```python
from build123d import *

# Parameters (mm, degrees)
SKETCH1_W           = 17
SKETCH1_H           = 30
BOSS_EXTRUDE1_DEPTH = 3
SKETCH2_W           = 3
SKETCH2_H           = 5
CUT_EXTRUDE1_DEPTH  = 3
SKETCH3_R           = 1.5
CUT_EXTRUDE2_DEPTH  = 3
FILLET1_R           = 3
SKETCH4_W           = 30
SKETCH4_H           = 30
BOSS_EXTRUDE2_DEPTH = 3
FILLET2_R           = 3
SKETCH5_R           = 2
CUT_EXTRUDE3_DEPTH  = 3
SKETCH6_W           = 3
SKETCH6_H           = 3
CUT_EXTRUDE4_DEPTH  = 10


with BuildPart() as part:
    # Sketch1 → Boss-Extrude1 (new body)
    with BuildSketch(Plane(origin=(0, 0, 0), x_dir=(1, 0, 0), z_dir=(0, 1, 0))):
        Rectangle(SKETCH1_W, SKETCH1_H)
    extrude(amount=BOSS_EXTRUDE1_DEPTH)

    # Sketch2 → Cut-Extrude1 (cut)
    with BuildSketch(Plane(origin=(0, 3, 0), x_dir=(1, 0, 0), z_dir=(0, 1, 0))):
        with Locations((7, 10)):
            Rectangle(SKETCH2_W, SKETCH2_H)
        with Locations((7, 0)):
            Rectangle(SKETCH2_W, SKETCH2_H)
        with Locations((7, -10)):
            Rectangle(SKETCH2_W, SKETCH2_H)
    extrude(amount=-CUT_EXTRUDE1_DEPTH, mode=Mode.SUBTRACT)

    # Sketch3 → Cut-Extrude2 (cut)
    with BuildSketch(Plane(origin=(0, 3, 0), x_dir=(1, 0, 0), z_dir=(0, 1, 0))):
        with Locations(Location((-4.5, 10, 0), (0, 0, 270))):
            Circle(SKETCH3_R)
        with Locations(Location((-4.5, -10, 0), (0, 0, 270))):
            Circle(SKETCH3_R)
    extrude(amount=-CUT_EXTRUDE2_DEPTH, mode=Mode.SUBTRACT)

    # Fillet1
    fillet1_edges = [part.edges().sort_by_distance(p)[0] for p in [
        (-8.5, 1.5, 15),
        (-8.5, 1.5, -15),
    ]]
    fillet(fillet1_edges, radius=FILLET1_R)

    # Sketch4 → Boss-Extrude2 (add)
    with BuildSketch(Plane(origin=(0, 3, 0), x_dir=(1, 0, 0), z_dir=(0, 1, 0))):
        with Locations((23.5, 0)):
            Rectangle(SKETCH4_W, SKETCH4_H)
    extrude(amount=-BOSS_EXTRUDE2_DEPTH)

    # Fillet2
    fillet2_edges = [part.edges().sort_by_distance(p)[0] for p in [
        (38.5, 1.5, 15),
        (38.5, 1.5, -15),
    ]]
    fillet(fillet2_edges, radius=FILLET2_R)

    # Sketch5 → Cut-Extrude3 (cut)
    with BuildSketch(Plane(origin=(0, 3, 0), x_dir=(1, 0, 0), z_dir=(0, 1, 0))):
        with Locations(Location((23.5, 0, 0), (0, 0, 270))):
            Circle(SKETCH5_R)
    extrude(amount=-CUT_EXTRUDE3_DEPTH, mode=Mode.SUBTRACT)

    # Sketch6 → Cut-Extrude4 (cut)
    with BuildSketch(Plane(origin=(0, 3, 0), x_dir=(1, 0, 0), z_dir=(0, 1, 0))):
        with Locations((13, 5)):
            Rectangle(SKETCH6_W, SKETCH6_H)
        with Locations((13, -5)):
            Rectangle(SKETCH6_W, SKETCH6_H)
    extrude(amount=-CUT_EXTRUDE4_DEPTH, mode=Mode.SUBTRACT)


solid = part.part
```
Input: part model. Units: mm. Frame: model coordinates. A direction names the side the tool comes from. Coordinates: 2 decimals unless noted, no trailing zeros. Write each loop counter-clockwise with the first axis right and the second up, starting at its lowest first coordinate (ties: lowest second). Pieces come first, ordered by that corner, then holes.
1) Pin query (flat end, axial travel): pin 1 Ø2.5 at (x, z) = (-4.5, 10) entering from +Y. Return the tip coordinate at first contact, or that it passes through.
2) Section D-D on z = 4.75. Output: boundary loops of the cut face in (x, y).
3) Mould query, pull axis Z, two halves, no side actions, for faces 3 (the flat face through (38.5, 2, 0)), 4 (the cylindrical face through (-4.43, 1.52, -11.5)), 5 (the flat face through (15, 2, -15)). Classes: pulls with the +Z half, pulls with the -Z half, needs draft (parallel to the pull), parting line crosses it, or undercut.
4) Section C-C on y = 0.85. State how many separate pieces and enclosed holes the cut face has, and give its area (3 significant figures).
5) Set-up query: faces 1 (the cylindrical face through (37.6, 1.48, -14.14)), 2 (the flat face through (5.5, 2, 10)). Return all of +Z, -Z, +X, -X, +Y, -Y with unobstructed straight access to the full face (end or side cutting, diameter ignored); none if empty.
6) Material intervals for line 1 along X through (y, z) = (0.8, -10); line 2 along X through (y, z) = (2.1, 0); line 3 along Z through (x, y) = (12.5, 2.9), sorted ascending.
7) Section A-A on z = 0. Output: boundary loops of the cut face in (x, y), and give its area (3 significant figures).
8) Section B-B on x = -4.5. Output: boundary loops of the cut face in (y, z).
Check result:
1. pin 1: passes through
2. outline: (-8.5, 0) - (11.5, 0) - (11.5, 3) - (-8.5, 3) - close; (14.5, 0) - (38.5, 0) - (38.5, 3) - (14.5, 3) - close
3. face 3: needs draft
3. face 4: undercut
3. face 5: pulls with the -Z half
4. separate pieces: 1
4. enclosed holes: 8
4. area: 1,310 mm2
5. face 1: -Z, +X, +Y, -Y
5. face 2: +Y, -Y
6. line 1: x = -8.5 to -6, -3 to 5.5, 8.5 to 38.5
6. line 2: x = -8.5 to 5.5, 8.5 to 21.5, 25.5 to 38.5
6. line 3: z = -15 to -6.5, -3.5 to 3.5, 6.5 to 15
7. outline: (-8.5, 0) - (5.5, 0) - (5.5, 3) - (-8.5, 3) - close; (8.5, 0) - (21.5, 0) - (21.5, 3) - (8.5, 3) - close; (25.5, 0) - (38.5, 0) - (38.5, 3) - (25.5, 3) - close
7. area: 120 mm2
8. outline: (0, -15) - (3, -15) - (3, -11.5) - (0, -11.5) - close; (0, -8.5) - (3, -8.5) - (3, 8.5) - (0, 8.5) - close; (0, 11.5) - (3, 11.5) - (3, 15) - (0, 15) - close
